Autodesk Inventor part; units mm, degrees
ref_plane "YZ Plane" through (0, 0, 0) normal (1, 0, 0) x (0, 1, 0)
ref_plane "XZ Plane" through (0, 0, 0) normal (0, 1, 0) x (-1, 0, 0)
ref_plane "XY Plane" through (0, 0, 0) normal (0, 0, 1) x (1, 0, 0)
sketch "Skizze1" plane through (0, 0, 0) normal (0, 1, 0) x (-1, 0, 0)
  line L0 (28.45, 17) -> (-28.45, 17)
  line L1 (-28.45, 17) -> (-28.45, -17)
  line L2 (-28.45, -17) -> (28.45, -17)
  line L3 (28.45, -17) -> (28.45, 17)
  line L4 (28.45, 17) -> (-28.45, -17) construction
  line L5 (-28.45, 17) -> (28.45, -17) construction
  point P0 (0, 0)
  dimension "d0" = 56.9
  dimension "d1" = 34
extrude "Extrusion1" add sketch "Skizze1" along normal blind 3
sketch "Skizze2" plane through (0, 3, 0) normal (0, 1, 0) x (1, 0, 0)
  line L0 (-6.15, -15.1) -> (6.15, -15.1)
  line L1 (6.15, -15.1) -> (6.15, 15.1)
  line L2 (6.15, 15.1) -> (-6.15, 15.1)
  line L3 (-6.15, 15.1) -> (-6.15, -15.1)
  line L4 (-6.15, -15.1) -> (6.15, 15.1) construction
  line L5 (6.15, -15.1) -> (-6.15, 15.1) construction
  line L6 (10.15, -15.1) -> (22.45, -15.1)
  line L7 (22.45, -15.1) -> (22.45, 15.1)
  line L8 (22.45, 15.1) -> (10.15, 15.1)
  line L9 (10.15, 15.1) -> (10.15, -15.1)
  line L10 (10.15, -15.1) -> (22.45, 15.1) construction
  line L11 (22.45, -15.1) -> (10.15, 15.1) construction
  line L12 (-22.45, -15.1) -> (-10.15, -15.1)
  line L13 (-10.15, -15.1) -> (-10.15, 15.1)
  line L14 (-10.15, 15.1) -> (-22.45, 15.1)
  line L15 (-22.45, 15.1) -> (-22.45, -15.1)
  line L16 (-22.45, -15.1) -> (-10.15, 15.1) construction
  line L17 (-10.15, -15.1) -> (-22.45, 15.1) construction
  line L18 (-28.45, 17) -> (-28.45, -17)
  line L19 (28.45, -17) -> (28.45, 17)
  point P0 (0, 0)
  point P1 (0, 0)
  point P2 (16.3, 0)
  point P3 (-16.3, 0)
  dimension "d4" = 12.3
  dimension "d5" = 30.2
  dimension "d6" = 12.3
  dimension "d7" = 30.2
  dimension "d8" = 12.3
  dimension "d9" = 30.2
  dimension "d10" = 4
  dimension "d11" = 4
  dimension "d12" = 6
  dimension "d13" = 6
extrude "Extrusion2" cut sketch "Skizze2" against normal blind 3
sketch "Skizze3" plane through (0, 3, 0) normal (0, 1, 0) x (1, 0, 0)
  line L0 (-25.65, 10) -> (25.65, 10)
  line L1 (25.65, 10) -> (25.65, -10)
  line L2 (25.65, -10) -> (-25.65, -10)
  line L3 (-25.65, -10) -> (-25.65, 10)
  line L4 (-25.65, 10) -> (25.65, -10) construction
  line L5 (25.65, 10) -> (-25.65, -10) construction
  line L6 (-25.65, 0) -> (25.65, 0)
  point P0 (0, 0)
  dimension "d16" = 51.3
  dimension "d17" = 20
hole "Bohrung1" at (-25.65, 3, 0) at (25.65, 3, 0) direction (0, -1, 0) diameter 2.4 end through all countersink diameter 4.4 countersink angle 90
fillet "Rundung1" radius 6 4 edges at (28.45, 1.5, 17) (28.45, 1.5, -17) (-28.45, 1.5, 17) (-28.45, 1.5, -17)
chamfer "Fase1" distance 1.5 angle 45 6 edges at (-6.15, 0, 0) (10.15, 0, 0) (6.15, 0, 0) (-10.15, 0, 0) (22.45, 0, 0) (-22.45, 0, 0)
properties part number "Wago2Din"
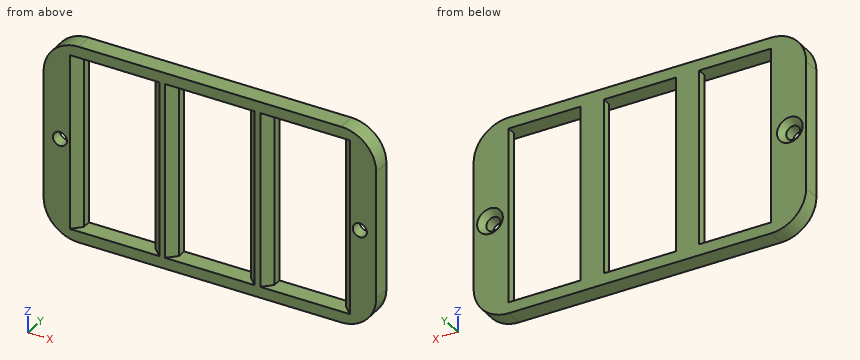
Input: part model. Units: mm. Frame: model coordinates. Coordinates: 2 decimals unless noted, no trailing zeros. Write each loop counter-clockwise with the first axis right and the second up, starting at its lowest first coordinate (ties: lowest second). Pieces come first, ordered by that corner, then holes. Notation, with made-up numbers: (-11.5, 30) - (33.5, 30) arc R15 ccw to (33.5, 46) - close; hole circle Ø11 at (33.25, -29). An arc over 180 degrees is marked (long way). Put each result on its own line as item: value. Start each with the question number.
1) Cut plane D-D (x = 25.65). Return the cut outline in (y, z).
2) Cut plane A-A (z = 0). State how many separate pieces and enclosed holes the cut face has, plus the area to 4 significant figures.
3) Ray query, L1, parallel to X at y = 2.95, z = 7; L2, parallel to X at y = 1.65, z = 0; L3, parallel to X at y = 0.8, z = 3. Return the intervals inside material, ascending.
4) Cut plane B-B (x = 15.5). Return the cut outline in (y, z), plus the area to 3 significant figures.
5) Cut plane C-C (z = 6). Return the cut outline in (x, y).
Resolved:
1. outline: (0, -16.08) - (3, -16.08) - (3, -2.2) - (2, -1.2) - (0, -1.2) - close; (0, 1.2) - (2, 1.2) - (3, 2.2) - (3, 16.08) - (0, 16.08) - close
2. separate pieces: 6
2. enclosed holes: 0
2. area: 36.85 mm2
3. L1: x = -28.45 to -22.45, -10.15 to -6.15, 6.15 to 10.15, 22.45 to 28.45
3. L2: x = -28.45 to -26.85, -24.45 to -22.45, -10.15 to -6.15, 6.15 to 10.15, 22.45 to 24.45, 26.85 to 28.45
3. L3: x = -28.45 to -23.15, -9.45 to -6.85, 6.85 to 9.45, 23.15 to 28.45
4. outline: (0, -17) - (3, -17) - (3, -15.1) - (0, -15.1) - close; (0, 15.1) - (3, 15.1) - (3, 17) - (0, 17) - close
4. area: 11.4 mm2
5. outline: (-28.45, 0) - (-23.95, 0) - (-22.45, 1.5) - (-22.45, 3) - (-28.45, 3) - close; (-10.15, 1.5) - (-8.65, 0) - (-7.65, 0) - (-6.15, 1.5) - (-6.15, 3) - (-10.15, 3) - close; (6.15, 1.5) - (7.65, 0) - (8.65, 0) - (10.15, 1.5) - (10.15, 3) - (6.15, 3) - close; (22.45, 1.5) - (23.95, 0) - (28.45, 0) - (28.45, 3) - (22.45, 3) - close
